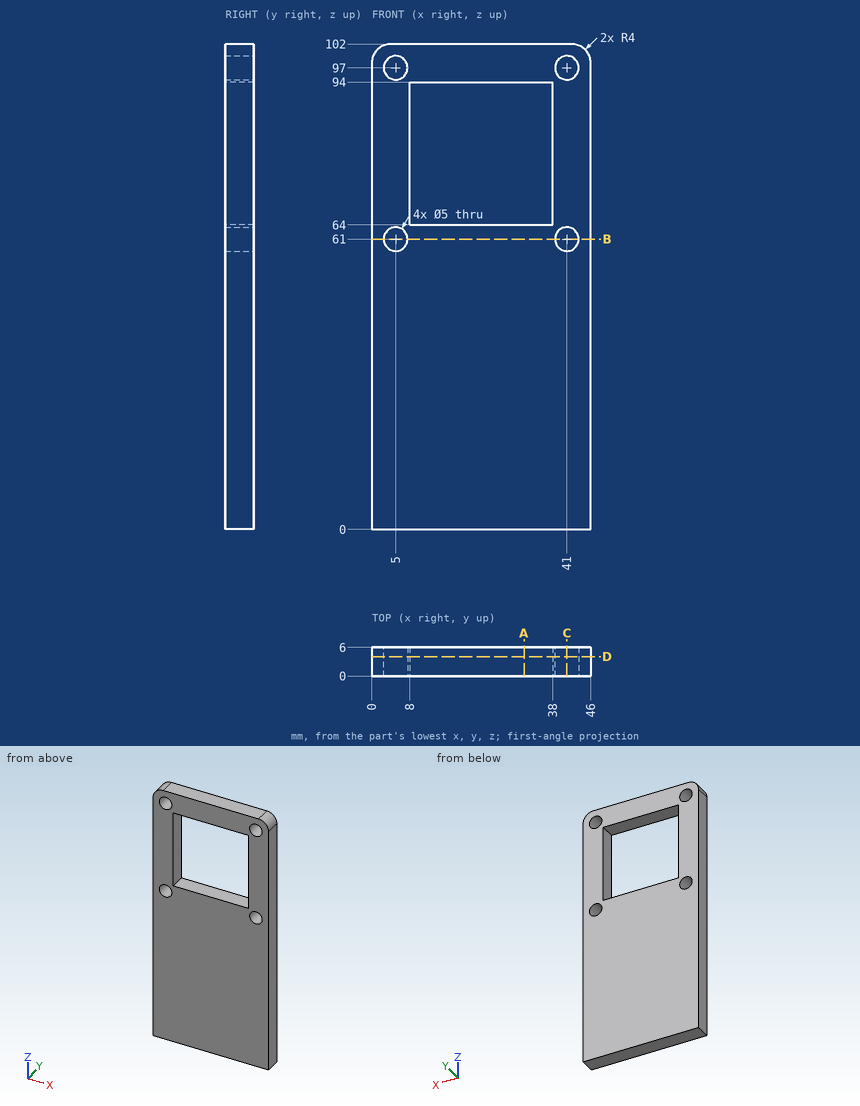
Answer from the drawing. Dimensions are ordinates in mm from the lowest x, y and z of the part. Coordinates: 2 decimals unless noted, no trailing zeros. Write each loop counter-clockwise with the first axis right and the second up, starting at its lowest first coordinate (ties: lowest second). Pieces come first, ordered by that corner, then holes. Notation, with made-up numbers: (16.5, 18.5) - (27.5, 18.5) arc R21 cw to (27.5, 54.5) - close; hole circle Ø2 at (67, 7). An arc over 180 degrees is marked (long way). Return JSON: item names as keys, results as strings.
1. The part is cut by section B-B on z = 61. Determine the outline of the cut face in (x, y).
Final values:
{"outline": "(0, 0) - (2.5, 0) - (2.5, 6) - (0, 6) - close; (7.5, 0) - (38.5, 0) - (38.5, 6) - (7.5, 6) - close; (43.5, 0) - (46, 0) - (46, 6) - (43.5, 6) - close"}
2. This flat-tipped pin is pushed along its axis until it touches: pin 1 Ø1.8 at (y, z) = (3.5, 83) entering from -X. Where does it stop, or does it pass through?
Final values:
{"pin 1": "x = 0"}
3. The part is cut by section D-D on y = 4.05. Determine the outline of the cut face in (x, z).
Final values:
{"outline": "(0, 0) - (46, 0) - (46, 98) arc R4 ccw to (42, 102) - (4, 102) arc R4 ccw to (0, 98) - close; hole circle Ø5 at (5, 61); hole circle Ø5 at (5, 97); hole (8, 64) - (38, 64) - (38, 94) - (8, 94) - close; hole circle Ø5 at (41, 61); hole circle Ø5 at (41, 97)"}
4. The part is cut by section A-A on x = 32. Determine the outline of the cut face in (y, z), then the cut area to 3 significant figures.
Final values:
{"outline": "(0, 0) - (6, 0) - (6, 64) - (0, 64) - close; (0, 94) - (6, 94) - (6, 102) - (0, 102) - close", "area": "432 mm^2"}
5. Consider line 1 along Z through (x, y) = (41, 3.65); line 2 along X through (y, z) = (1.35, 93.5); line 3 along X through (y, z) = (4.2, 97). Determine where each line is inside the solid, lowest interval first.
Final values:
{"line 1": "0 to 58.5, 63.5 to 94.5, 99.5 to 102", "line 2": "0 to 8, 38 to 46", "line 3": "0 to 2.5, 7.5 to 38.5, 43.5 to 46"}
6. The part is cut by section C-C on x = 41. Determine the outline of the cut face in (y, z), then the cut area to 3 significant figures.
Final values:
{"outline": "(0, 0) - (6, 0) - (6, 58.5) - (0, 58.5) - close; (0, 63.5) - (6, 63.5) - (6, 94.5) - (0, 94.5) - close; (0, 99.5) - (6, 99.5) - (6, 102) - (0, 102) - close", "area": "552 mm^2"}
